from build123d import *

# Parameters (mm, degrees)
SKETCH1_W          = 150
SKETCH1_H          = 30
SKETCH1_R          = 3.5
SKETCH1_R_2        = 3
BASE_FLANGE1_DEPTH = 4
FILLET1_R          = 1


# Sheet-metal steps are written as plain solids
with BuildPart() as part:
    # Sketch1 → Base-Flange1 (new body)
    with BuildSketch(Plane.XY):
        Rectangle(SKETCH1_W, SKETCH1_H)
        with Locations((25, 0)):
            Circle(SKETCH1_R, mode=Mode.SUBTRACT)
        with Locations((-25, 0)):
            Circle(SKETCH1_R, mode=Mode.SUBTRACT)
        with Locations((65, -10)):
            Circle(SKETCH1_R_2, mode=Mode.SUBTRACT)
        with Locations((65, 10)):
            Circle(SKETCH1_R_2, mode=Mode.SUBTRACT)
        with Locations((-65, -10)):
            Circle(SKETCH1_R_2, mode=Mode.SUBTRACT)
        with Locations((-65, 10)):
            Circle(SKETCH1_R_2, mode=Mode.SUBTRACT)
    extrude(amount=-BASE_FLANGE1_DEPTH)

    # Fillet1
    fillet1_edges = [part.edges().sort_by_distance(p)[0] for p in [
        (-75, 15, -2),
        (75, 15, -2),
        (75, -15, -2),
        (-75, -15, -2),
    ]]
    fillet(fillet1_edges, radius=FILLET1_R)


solid = part.part
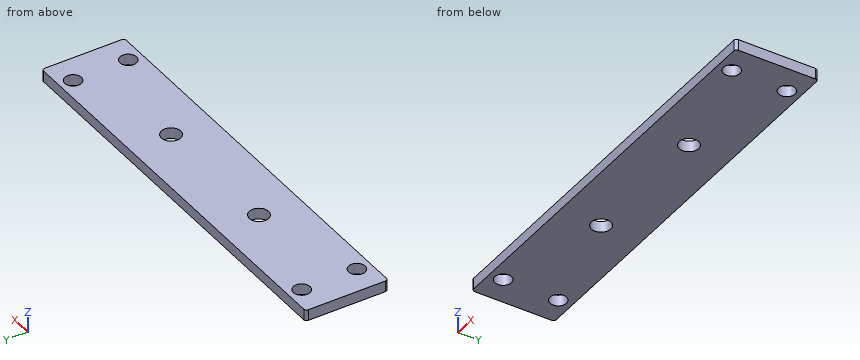
Geometry: final body of the model. Coordinates: model frame, mm. Round coordinates to 2 decimals unless told otherwise and drop trailing zeros. Loops run counter-clockwise (first coordinate to the right, second up) from the corner with the lowest first, then second, coordinate; pieces in that order, holes last.
Q1. Section C-C on z = -2.7. Return loops of the section in (x, y), plus the area to 3 significant figures.
Q2. Section A-A on y = 0. Return loops of the section in (x, z), plus the area to 3 significant figures.
Q3. Section B-B on x = 25. Return loops of the section in (y, z).
Q4. Material intervals for L1, parallel to Y at x = 65, z = -3.2; L2, parallel to Y at x = -25, z = -0.95; L3, parallel to X at y = -8, z = -1.05, sorted ascending.
Q5. Pin query (flat end, axial travel): P1, Ø3.5, axis at x = -65, y = 10, coming from the +Z side; P2, Ø7, axis at x = 65, y = -10, coming from the +Z side. Return the tip coordinate at first contact, or that it passes through.
Q6. Section D-D on x = 65. Return loops of the section in (y, z).
Evaluation:
1. outline: (-75, -14) arc R1 ccw to (-74, -15) - (74, -15) arc R1 ccw to (75, -14) - (75, 14) arc R1 ccw to (74, 15) - (-74, 15) arc R1 ccw to (-75, 14) - close; hole circle Ø6 at (-65, -10); hole circle Ø6 at (-65, 10); hole circle Ø7 at (-25, 0); hole circle Ø7 at (25, 0); hole circle Ø6 at (65, -10); hole circle Ø6 at (65, 10)
1. area: 4,310 mm2
2. outline: (-75, -4) - (-28.5, -4) - (-28.5, 0) - (-75, 0) - close; (-21.5, -4) - (21.5, -4) - (21.5, 0) - (-21.5, 0) - close; (28.5, -4) - (75, -4) - (75, 0) - (28.5, 0) - close
2. area: 544 mm2
3. outline: (-15, -4) - (-3.5, -4) - (-3.5, 0) - (-15, 0) - close; (3.5, -4) - (15, -4) - (15, 0) - (3.5, 0) - close
4. L1: y = -15 to -13, -7 to 7, 13 to 15
4. L2: y = -15 to -3.5, 3.5 to 15
4. L3: x = -75 to -67.24, -62.76 to 62.76, 67.24 to 75
5. P1: passes through
5. P2: stops at z = 0
6. outline: (-15, -4) - (-13, -4) - (-13, 0) - (-15, 0) - close; (-7, -4) - (7, -4) - (7, 0) - (-7, 0) - close; (13, -4) - (15, -4) - (15, 0) - (13, 0) - close
